Check sheet for the modelled part. Datum: model origin and axes. Units: mm. Face numbers are marked on the shaded views. A direction names the side the tool comes from. Round coordinates to 2 decimals unless told otherwise and drop trailing zeros. Write each loop counter-clockwise with the first axis right and the second up, starting at its lowest first coordinate (ties: lowest second). Pieces come first, ordered by that corner, then holes. Notation, with made-up numbers: (7.25, -8) - (34.25, -8) arc R24 cw to (34.25, 31) - close; hole circle Ø1 at (30.5, 16). An arc over 180 degrees is marked (long way). Answer as a JSON object with one key per item and string values. Group by question number.
Item 1: Release check for a two-part mould opening along Z. For the marked faces 3, 4 and 5 record: pulls with the +Z half, pulls with the -Z half, needs draft (parallel to the pull), parting line crosses it, or undercut.
Item 2: Sectioned sample at A-A on y = 1.5. Record the boundary of the cut face in (x, z).
Item 3: Thickness scan on line 1 (X direction, y = 3.15, z = 0); line 2 (Y direction, x = 0.25, z = 1.75). Record the ranges inside material, lowest first.
Item 4: Gauge pin test, flat ends, axial feed: P1, Ø5, axis at y = 6, z = 4.5, coming from the -X side; P2, Ø2.5, axis at x = 1, z = -1, coming from the +Y side; P3, Ø3, axis at x = 3, z = -4.5, coming from the -Y side. Record the tip position at first contact, or that the pin passes through.
Item 5: Set-up check for the marked faces 1 and 2: record each of +Z, -Z, +X, -X, +Y, -Y from which the full face is reachable in a straight line by a thin tool's end or side.
Item 6: Sectioned sample at B-B on y = 11.25. Record the boundary of the cut face in (x, z).
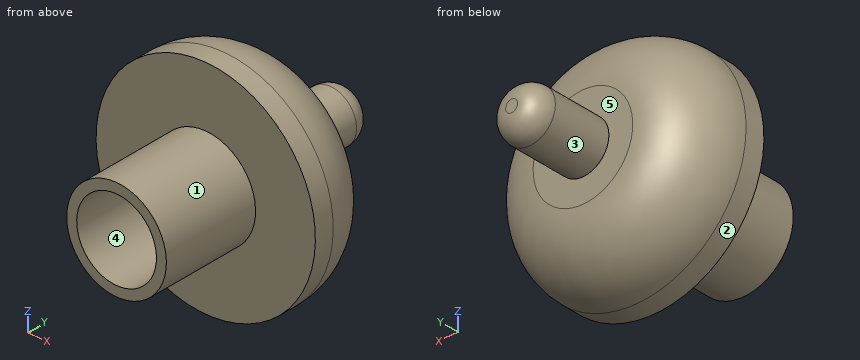
```python
from build123d import *

# Parameters (mm, degrees)
IZIM1_R                     = 2.5
IZIM1_R_2                   = 2
Y_KSEKLIK_EKSTR_ZYON1_DEPTH = 9
IZIM2_R                     = 5.5
Y_KSEKLIK_EKSTR_ZYON2_DEPTH = 4
RADYUS1_R                   = 3
IZIM3_R                     = 1.300236586
Y_KSEKLIK_EKSTR_ZYON3_DEPTH = 4
RADYUS2_R                   = 1


with BuildPart() as part:
    # izim1 → Y_kseklik-Ekstr_zyon1 (new body)
    with BuildSketch(Plane(origin=(0, 0, 0), x_dir=(1, 0, 0), z_dir=(0, 1, 0))):
        with Locations(Location((0, 0, 0), (0, 0, 270))):
            Circle(IZIM1_R)
        with Locations(Location((0, 0, 0), (0, 0, 270))):
            Circle(IZIM1_R_2, mode=Mode.SUBTRACT)
    extrude(amount=Y_KSEKLIK_EKSTR_ZYON1_DEPTH)



with BuildPart() as body_2:
    # izim2 → Y_kseklik-Ekstr_zyon2 (new body)
    with BuildSketch(Plane(origin=(0, 9, 0), x_dir=(1, 0, 0), z_dir=(0, 1, 0))):
        with Locations(Location((0, 0, 0), (0, 0, 270))):
            Circle(IZIM2_R)
    extrude(amount=-Y_KSEKLIK_EKSTR_ZYON2_DEPTH)

    # Radyus1
    radyus1_edges = [body_2.edges().sort_by_distance(p)[0] for p in [
        (0, 9, -5.5),
    ]]
    fillet(radyus1_edges, radius=RADYUS1_R)


with BuildPart() as part_1:
    add(part.part)

    add(body_2.part)  # Y_kseklik-Ekstr_zyon3 merges body 2
    # izim3 → Y_kseklik-Ekstr_zyon3 (add)
    with BuildSketch(Plane(origin=(0, 9, 0), x_dir=(1, 0, 0), z_dir=(0, 1, 0))):
        with Locations(Location((0, 0, 0), (0, 0, 270))):
            Circle(IZIM3_R)
    extrude(amount=Y_KSEKLIK_EKSTR_ZYON3_DEPTH)

    # Radyus2
    radyus2_edges = [part_1.edges().sort_by_distance(p)[0] for p in [
        (0, 13, -1.300236586),
    ]]
    fillet(radyus2_edges, radius=RADYUS2_R)


solid = part_1.part
```
Completed:
{
 "1": {"face 3": "parting line crosses it", "face 4": "undercut", "face 5": "needs draft"},
 "2": {"outline": "circle Ø5 at (0, 0); hole circle Ø4 at (0, 0)"},
 "3": {"line 1": "-2.5 to -2, 2 to 2.5", "line 2": "5 to 9"},
 "4": {"P1": "x = -5.12", "P2": "y = 13", "P3": "y = 5"},
 "5": {"face 1": "-Y", "face 2": "+Y, -Y"},
 "6": {"outline": "circle Ø2.6 at (0, 0)"}
}
